from build123d import *

# Parameters (mm, degrees)
SKETCH1_R           = 2
SKETCH1_R_2         = 1.6
BOSS_EXTRUDE1_DEPTH = 3.5


with BuildPart() as part:
    # Sketch1 → Boss-Extrude1 (new body)
    with BuildSketch(Plane(origin=(0, 0, 0), x_dir=(1, 0, 0), z_dir=(0, 1, 0))):
        with BuildLine():
            Line((33.5, 28), (33.5, 5))
            Line((33.5, 5), (50, 5))
            ThreePointArc((50, 5), (55, 0), (50, -5))
            Line((50, -5), (33.5, -5))
            Line((33.5, -5), (33.5, -28))
            ThreePointArc((33.5, -28), (29.5, -32), (25.5, -28))
            Line((25.5, -28), (25.5, -5))
            Line((25.5, -5), (-39.5, -5))
            Line((-39.5, -5), (-39.5, -28))
            ThreePointArc((-39.5, -28), (-43.5, -32), (-47.5, -28))
            Line((-47.5, -28), (-47.5, -5))
            Line((-47.5, -5), (-51.5, -5))
            ThreePointArc((-51.5, -5), (-56.5, 0), (-51.5, 5))
            Line((-51.5, 5), (-47.5, 5))
            Line((-47.5, 5), (-47.5, 28))
            ThreePointArc((-47.5, 28), (-43.5, 32), (-39.5, 28))
            Line((-39.5, 28), (-39.5, 5))
            Line((-39.5, 5), (25.5, 5))
            Line((25.5, 5), (25.5, 28))
            ThreePointArc((25.5, 28), (29.5, 32), (33.5, 28))
        make_face()
        with Locations((50, 0)):
            Circle(SKETCH1_R, mode=Mode.SUBTRACT)
        with Locations((-51.5, 0)):
            Circle(SKETCH1_R, mode=Mode.SUBTRACT)
        with Locations((29.5, 28)):
            Circle(SKETCH1_R_2, mode=Mode.SUBTRACT)
        with Locations((-43.5, 28)):
            Circle(SKETCH1_R_2, mode=Mode.SUBTRACT)
        with Locations((-43.5, -28)):
            Circle(SKETCH1_R_2, mode=Mode.SUBTRACT)
        with Locations((29.5, -28)):
            Circle(SKETCH1_R_2, mode=Mode.SUBTRACT)
    extrude(amount=BOSS_EXTRUDE1_DEPTH)


solid = part.part
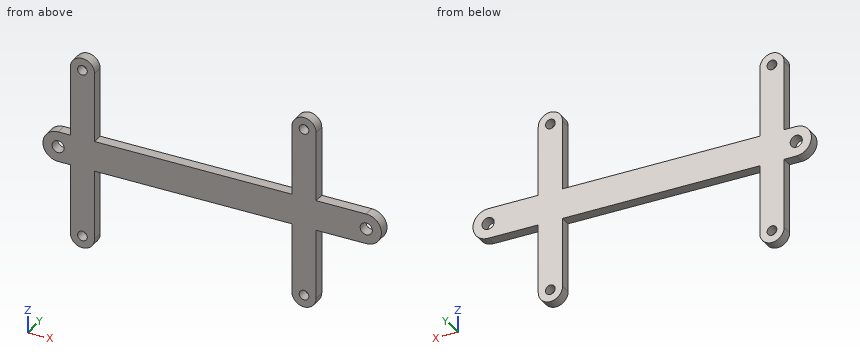
Could you check a few things on this model? Use its own coordinates, in mm. Give positions to 0.01 mm unless a question says otherwise; leave off trailing zeros. Order: outer loops, then holes, each group sorted by start corner. A loop starts at its lowest first (then second) coordinate and runs counter-clockwise, first axis right, second up.
Item 1: I need wall thicknesses on line 1 (X direction, y = 1.1, z = 28); line 2 (X direction, y = 1.3, z = 0); line 3 (Z direction, x = 29.5, y = 2.4). Which ranges of each line are inside material? Lowest first, please.
Item 2: I'm going to push flat-ended pins straight in: pin 1 (1 mm diameter, centred on y = 2.5, z = 13.5, fed in from +X); pin 2 (2 mm diameter, centred on x = -42, y = 2, fed in from -Z); pin 3 (5 mm diameter, centred on x = 50, z = 0, fed in from +Y); pin 4 (1.8 mm diameter, centred on x = -49.5, y = 2, fed in from +Z). Where does each tip first touch, or does it pass through?
Item 3: If we section it at A-A, the plane x = 29.5: Write out the boundary of the cut face in (y, z).
Item 4: If we section it at C-C, the plane z = 0: Write out the boundary of the cut face in (x, y).
Item 5: If we section it at D-D, the plane x = -2.5: Write out the boundary of the cut face in (y, z).
Item 6: If we section it at B-B, the plane z = 21: Write out the boundary of the cut face in (x, y), plus the area to 3 significant figures.
Values:
1. line 1: x = -47.5 to -45.1, -41.9 to -39.5, 25.5 to 27.9, 31.1 to 33.5
1. line 2: x = -56.5 to -53.5, -49.5 to 48, 52 to 55
1. line 3: z = -32 to -29.6, -26.4 to 26.4, 29.6 to 32
2. pin 1: stops at x = 33.5
2. pin 2: stops at z = -31.97
2. pin 3: stops at y = 3.5
2. pin 4: stops at z = 5
3. outline: (0, -32) - (3.5, -32) - (3.5, -29.6) - (0, -29.6) - close; (0, -26.4) - (3.5, -26.4) - (3.5, 26.4) - (0, 26.4) - close; (0, 29.6) - (3.5, 29.6) - (3.5, 32) - (0, 32) - close
4. outline: (-56.5, 0) - (-53.5, 0) - (-53.5, 3.5) - (-56.5, 3.5) - close; (-49.5, 0) - (48, 0) - (48, 3.5) - (-49.5, 3.5) - close; (52, 0) - (55, 0) - (55, 3.5) - (52, 3.5) - close
5. outline: (0, -5) - (3.5, -5) - (3.5, 5) - (0, 5) - close
6. outline: (-47.5, 0) - (-39.5, 0) - (-39.5, 3.5) - (-47.5, 3.5) - close; (25.5, 0) - (33.5, 0) - (33.5, 3.5) - (25.5, 3.5) - close
6. area: 56.0 mm2
